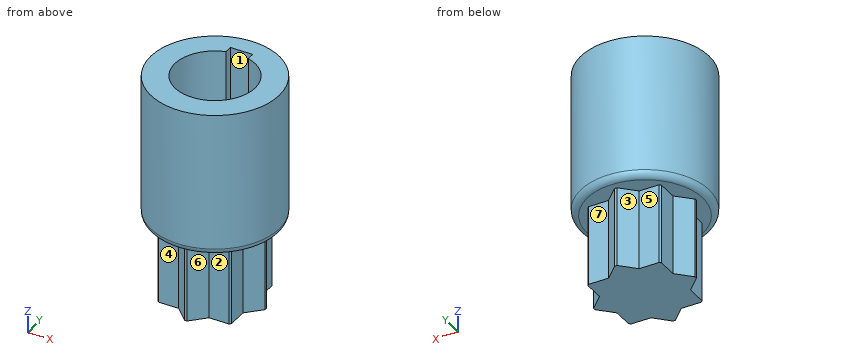
```python
from build123d import *

# Parameters (mm, degrees)
BOSS_EXTRUDE1_DEPTH = 50
SKETCH2_R           = 40
BOSS_EXTRUDE2_DEPTH = 90
SKETCH3_R           = 25
CUT_EXTRUDE1_DEPTH  = 67
SKETCH4_W           = 14
SKETCH4_H           = 28.8
CUT_EXTRUDE2_DEPTH  = 65
FILLET1_R           = 4
CHAMFER1_SIZE       = 0.5


with BuildPart() as part:
    # Sketch1 → Boss-Extrude1 (new body)
    with BuildSketch(Plane.XY):
        Polygon((0.707106781, -31.819805153), (9.526911935, -23), (22, -23), (23, -22), (23, -9.526911935), (31.819805153, -0.707106781), (31.819805153, 0.707106781), (23, 9.526911935), (23, 22), (22, 23), (9.526911935, 23), (0.707106781, 31.819805153), (-0.707106781, 31.819805153), (-9.526911935, 23), (-22, 23), (-23, 22), (-23, 9.526911935), (-31.819805153, 0.707106781), (-31.819805153, -0.707106781), (-23, -9.526911935), (-23, -22), (-22, -23), (-9.526911935, -23), (-0.707106781, -31.819805153), align=None)
    extrude(amount=BOSS_EXTRUDE1_DEPTH)

    # Sketch2 → Boss-Extrude2 (add)
    with BuildSketch(Plane.XY.offset(50)):
        with Locations(Location((0, 0, 0), (0, 0, 180))):
            Circle(SKETCH2_R)
    extrude(amount=BOSS_EXTRUDE2_DEPTH)

    # Sketch3 → Cut-Extrude1 (cut)
    with BuildSketch(Plane.XY.offset(140)):
        Circle(SKETCH3_R)
    extrude(amount=-CUT_EXTRUDE1_DEPTH, mode=Mode.SUBTRACT)

    # Sketch4 → Cut-Extrude2 (cut)
    with BuildSketch(Plane.XY.offset(140)):
        with Locations((0, 14.4)):
            Rectangle(SKETCH4_W, SKETCH4_H)
    extrude(amount=-CUT_EXTRUDE2_DEPTH, mode=Mode.SUBTRACT)

    # Fillet1
    fillet1_edges = [part.edges().sort_by_distance(p)[0] for p in [
        (40, 0, 50),
    ]]
    fillet(fillet1_edges, radius=FILLET1_R)

    # Chamfer1
    chamfer1_edges = [part.edges().sort_by_distance(p)[0] for p in [
        (-25, 0, 73),
    ]]
    chamfer(chamfer1_edges, length=CHAMFER1_SIZE)


solid = part.part
```
Check sheet for the modelled part. Datum: model origin and axes. Units: mm. Face numbers are marked on the shaded views. A direction names the side the tool comes from. Round coordinates to 2 decimals unless told otherwise and drop trailing zeros. Order: outer loops, then holes, each group sorted by start corner. A loop starts at its lowest first (then second) coordinate and runs counter-clockwise, first axis right, second up. Notation, with made-up numbers: M 28.25,14.25 L 62.25,14.25 A23 ccw 62.25,46.25 Z; hole C 82,35 d4. An arc over 180 degrees is marked long. Answer in a Markdown table with one row per item.
(1) Section check B-B on z = 21. Record the boundary of the cut face in (x, y), plus the area to 3 significant figures.
Findings:
| item | result |
|---|---|
| outline | M -31.82,-0.71 L -23,-9.53 L -23,-22 L -22,-23 L -9.53,-23 L -0.71,-31.82 L 0.71,-31.82 L 9.53,-23 L 22,-23 L 23,-22 L 23,-9.53 L 31.82,-0.71 L 31.82,0.71 L 23,9.53 L 23,22 L 22,23 L 9.53,23 L 0.71,31.82 L -0.71,31.82 L -9.53,23 L -22,23 L -23,22 L -23,9.53 L -31.82,0.71 Z |
| area | 2,480 mm^2 |
(2) Gauge pin test, flat ends, axial feed: pin 1 (10 mm diameter, centred on x = 18.5, z = 30.5, fed in from -Y); pin 2 (10 mm diameter, centred on y = 17.5, z = 16, fed in from -X); pin 3 (1.4 mm diameter, centred on x = 2, y = 26.5, fed in from +Z). Record the tip position at first contact, or that the pin passes through.
Findings:
| item | result |
|---|---|
| pin 1 | stops at y = -23 |
| pin 2 | stops at x = -23 |
| pin 3 | stops at z = 75 |
(3) Draft check along Y on the marked faces 1, 2 and 3. Enter one of: +Y half, -Y half, draft (parallel to the pull), parting line (faces both ways), or undercut.
Findings:
| item | result |
|---|---|
| face 1 | undercut |
| face 2 | -Y half |
| face 3 | +Y half |
(4) Set-up check for the marked faces 4, 5, 6 and 7: record each of +Z, -Z, +X, -X, +Y, -Y from which the full face is reachable in a straight line by a thin tool's end or side.
Findings:
| item | result |
|---|---|
| face 4 | -Z, -X, -Y |
| face 5 | -Z, -X, +Y |
| face 6 | -Z, +X, -Y |
| face 7 | -Z, +X, +Y |
(5) Section check A-A on z = 117.5. Record the boundary of the cut face in (x, y), plus the area to 3 significant figures.
Findings:
| item | result |
|---|---|
| outline | C 0,0 d80; hole M -7,24 A25 ccw long 7,24 L 7,28.8 L -7,28.8 Z |
| area | 3,010 mm^2 |
(6) Material ranges on line 1 along Y through (x, z) = (0, 110); line 2 along X through (y, z) = (1, 102); line 3 along Z through (x, y) = (5, -16), recorded low to high. Write a range as from..to.
Findings:
| item | result |
|---|---|
| line 1 | y = -40..-25, 28.8..40 |
| line 2 | x = -39.99..-24.98, 24.98..39.99 |
| line 3 | z = 0..73 |
